Can you work these out from the model? Positions are in its coordinate system, mm. A direction names the side the tool comes from. Round coordinates to 2 decimals unless told otherwise and drop trailing zeros. Loops run counter-clockwise (first coordinate to the right, second up) from the corner with the lowest first, then second, coordinate; pieces in that order, holes last. Notation, with made-up numbers: M 45,1.25 L 74,1.25 A8 cw 74,15.25 Z; hole C 13.5,17 d1. An arc over 180 degrees is marked long. Return JSON: item names as keys, results as strings.
```python
from build123d import *

# Parameters (mm, degrees)
SKETCH3_R               = 14
SKETCH3_R_2             = 6.35
SKETCH3_R_3             = 20
SKETCH3_R_4             = 9.5
BOSS_EXTRUDE6_DEPTH     = 26.5
CUT_EXTRUDE5_START      = 7
SKETCH7_W               = 38
SKETCH7_H               = 71.155333985
CUT_EXTRUDE5_DEPTH      = 12.5
CUT_EXTRUDE6_DEPTH      = 93.278112248
CUT_EXTRUDE6_DEPTH_BACK = 6
CUT_EXTRUDE8_DEPTH      = 93.278112248
CUT_EXTRUDE8_DEPTH_BACK = 6
CUT_EXTRUDE10_DEPTH     = 5
CUT_EXTRUDE10_TAPER     = 5
CUT_EXTRUDE11_DEPTH     = 5
CUT_EXTRUDE11_DRAFT     = -5


with BuildPart() as part:
    # Sketch3 → Boss-Extrude6 (new body)
    # profile 1 of 3: a face of its own
    with BuildSketch(Plane.XY):
        with BuildLine():
            ThreePointArc((0.870489571, 49), (-12.127650844, 35.035893248), (-26.986121482, 47.001417973))
            Line((-26.986121482, 47.001417973), (-19.795158647, -2.855117182))
            ThreePointArc((-19.795158647, -2.855117182), (-1.431227978, 19.948723931), (20, 0))
            ThreePointArc((20, 0), (14.142135624, -14.142135624), (0, -20))
            Line((0, -20), (62, -20))
            Line((62, -20), (62, -8.5))
            Line((62, -8.5), (40, -8.5))
            ThreePointArc((40, -8.5), (33.5, -2), (40, 4.5))
            Line((40, 4.5), (62, 4.5))
            Line((62, 4.5), (62, 16))
            ThreePointArc((62, 16), (24.979840385, 26.107737846), (-0.421043253, 54.873232673))
            ThreePointArc((-0.421043253, 54.873232673), (0.543794593, 52.006780632), (0.870489571, 49))
        make_face()
    # profile 2 of 3: a face of its own
    with BuildSketch(Plane.XY):
        with Locations((-13.129510429, 49)):
            Circle(SKETCH3_R)
        with Locations((-13.129510429, 49)):
            Circle(SKETCH3_R_2, mode=Mode.SUBTRACT)
    # profile 3 of 3: a face of its own
    with BuildSketch(Plane.XY):
        Circle(SKETCH3_R_3)
        Circle(SKETCH3_R_4, mode=Mode.SUBTRACT)
    extrude(amount=BOSS_EXTRUDE6_DEPTH)

    # Sketch7 → Cut-Extrude5 (cut)
    with BuildSketch(Plane.XY.offset(CUT_EXTRUDE5_START)):
        with Locations((43, 15.577666993)):
            Rectangle(SKETCH7_W, SKETCH7_H)
    extrude(amount=CUT_EXTRUDE5_DEPTH, mode=Mode.SUBTRACT)

    # Sketch8 → Cut-Extrude6 (cut, two sides: drawn at the far end of the back side and taken through both)
    with BuildSketch(Plane.XY.offset(26.5).offset(-CUT_EXTRUDE6_DEPTH_BACK)):
        with BuildLine():
            Line((-191.908254211, 170.560932392), (-25.15238927, 34.287747135))
            ThreePointArc((-25.15238927, 34.287747135), (-9.427586496, 30.364127088), (3.603690102, 40))
            Line((3.603690102, 40), (9.001095845, 40))
            Line((9.001095845, 40), (224.356382551, 40))
            Line((224.356382551, 40), (353.256649812, 450.969973536))
            Line((353.256649812, 450.969973536), (-63.007986949, 581.530905928))
            Line((-63.007986949, 581.530905928), (-191.908254211, 170.560932392))
        make_face()
    extrude(amount=CUT_EXTRUDE6_DEPTH + CUT_EXTRUDE6_DEPTH_BACK, mode=Mode.SUBTRACT)

    # Sketch9 → Cut-Extrude8 (cut, two sides: drawn at the far end of the back side and taken through both)
    with BuildSketch(Plane(origin=(0, 0, 0), x_dir=(-1, 0, 0), z_dir=(0, 0, -1)).offset(-CUT_EXTRUDE8_DEPTH_BACK)):
        with BuildLine():
            Line((191.908254211, 170.560932392), (25.15238927, 34.287747135))
            ThreePointArc((25.15238927, 34.287747135), (9.427586496, 30.364127088), (-3.603690102, 40))
            Line((-3.603690102, 40), (-9.001095845, 40))
            Line((-9.001095845, 40), (-224.356382551, 40))
            Line((-224.356382551, 40), (-353.256649812, 450.969973536))
            Line((-353.256649812, 450.969973536), (63.007986949, 581.530905928))
            Line((63.007986949, 581.530905928), (191.908254211, 170.560932392))
        make_face()
    extrude(amount=CUT_EXTRUDE8_DEPTH + CUT_EXTRUDE8_DEPTH_BACK, mode=Mode.SUBTRACT)

    # Sketch11 → Cut-Extrude10 (cut)
    with BuildSketch(Plane.XY):
        with BuildLine():
            Line((8.074790236, 38), (4.759033391, 38))
            ThreePointArc((4.759033391, 38), (-7.381776563, 28.801892282), (-22.54639569, 30.229750349))
            Line((-22.54639569, 30.229750349), (-17.815642783, -2.569605464))
            ThreePointArc((-17.815642783, -2.569605464), (-11.784462263, -13.606118079), (0, -18))
            Line((0, -18), (60, -18))
            Line((60, -18), (60, -10.5))
            Line((60, -10.5), (40, -10.5))
            ThreePointArc((40, -10.5), (31.5, -2), (40, 6.5))
            Line((40, 6.5), (60, 6.5))
            Line((60, 6.5), (60, 13.981994332))
            ThreePointArc((60, 13.981994332), (31.430822369, 20.355773383), (8.074790236, 38))
        make_face()
    extrude(amount=CUT_EXTRUDE10_DEPTH, taper=CUT_EXTRUDE10_TAPER, mode=Mode.SUBTRACT)


with BuildPart() as cut_extrude11_tool:
    # Sketch12 → Cut-Extrude11 (with draft: the straight prism first)
    with BuildSketch(Plane.XY.offset(26.5)):
        with BuildLine():
            Line((8.074790236, 38), (4.759033391, 38))
            ThreePointArc((4.759033391, 38), (-7.381776563, 28.801892282), (-22.54639569, 30.229750349))
            Line((-22.54639569, 30.229750349), (-17.815642783, -2.569605464))
            ThreePointArc((-17.815642783, -2.569605464), (-11.784462263, -13.606118079), (0, -18))
            Line((0, -18), (60, -18))
            Line((60, -18), (60, -10.5))
            Line((60, -10.5), (40, -10.5))
            ThreePointArc((40, -10.5), (31.5, -2), (40, 6.5))
            Line((40, 6.5), (60, 6.5))
            Line((60, 6.5), (60, 13.981994332))
            ThreePointArc((60, 13.981994332), (31.430822369, 20.355773383), (8.074790236, 38))
        make_face()
    extrude(amount=-CUT_EXTRUDE11_DEPTH)
    # Cut-Extrude11: the draft: its side faces are tilted about the plane it starts from
    cut_extrude11_sides = [cut_extrude11_tool.faces().sort_by_distance(p)[0] for p in [
        (31.430822369, 20.355773383, 24),
        (6.416911814, 38, 24),
        (-7.381776563, 28.801892282, 24),
        (-20.181019237, 13.830072443, 24),
        (-11.784462263, -13.606118079, 24),
        (30, -18, 24),
        (60, -14.25, 24),
        (50, -10.5, 24),
        (31.5, -2, 24),
        (50, 6.5, 24),
        (60, 10.240997166, 24),
    ]]
    draft(cut_extrude11_sides, Plane.XY.offset(26.5), CUT_EXTRUDE11_DRAFT)


with BuildPart() as part_1:
    add(part.part)

    # Cut-Extrude11: cut by cut_extrude11_tool
    add(cut_extrude11_tool.part, mode=Mode.SUBTRACT)


solid = part_1.part
```
Q1. Thinking about a two-plate mould opening in Y: for faces 1 (the flat face through (-23.44, 22.42, 13.06)), 2 (the conical face through (-7.11, 28.65, 2.54)), 3 (the flat face through (34, 4, 7)), which applies, pulls with the +Y half, pulls with the -Y half, needs draft (parallel to the pull), parting line crosses it, or undercut?
Results:
{"face 1": "pulls with the -Y half", "face 2": "undercut", "face 3": "needs draft"}
Q2. Suppose I cut it at A-A, the plane z = 17.75. Please give me the cut outline in (x, y).
Results:
{"outline": "M -26.99,47 L -19.8,-2.86 A20 ccw 0,-20 L 24,-20 L 24,26.73 A67 cw -0.42,54.87 A14 ccw Z; hole C -13.13,49 d12.7; hole C 0,0 d19"}
Q3. Suppose I cut it at C-C, the plane z = 23.75. Please give me the cut outline in (x, y), plus the area to 3 significant figures.
Results:
{"outline": "M -25.15,34.29 L -19.8,-2.86 A20 ccw 0,-20 L 62,-20 L 62,-8.5 L 40,-8.5 A6.5 cw 40,4.5 L 62,4.5 L 62,16 A67 cw 9,40 L 3.6,40 A19 cw Z; hole M -22.24,29.81 L -17.58,-2.54 A17.76 ccw 0,-17.76 L 59.76,-17.76 L 59.76,-10.74 L 40,-10.74 A8.74 cw 40,6.74 L 59.76,6.74 L 59.76,13.74 A69.24 cw 7.96,37.76 L 4.89,37.76 A21.24 cw Z", "area": "679 mm2"}
Q4. Suppose I cut it at D-D, the plane x = 50. State how many separate pieces and enclosed holes the cut face has, plus the area to 3 significant figures.
Results:
{"separate pieces": "4", "enclosed holes": "0", "area": "184 mm2"}
Q5. I'm going to push flat-ended pins straight in: pin 1 Ø10 at (x, y) = (-17, 47.5) entering from -Z; pin 2 Ø1.6 at (x, z) = (7.5, 24) entering from +Y; pin 3 Ø6 at (y, z) = (12.5, 15) entering from +X; pin 4 Ø11.5 at (x, y) = (34.5, 0) entering from +Z. Where does each tip first touch, or does it pass through?
Results:
{"pin 1": "stops at z = 6", "pin 2": "stops at y = 40", "pin 3": "stops at x = 24", "pin 4": "stops at z = 26.5"}
Q6. On a 3-axis mill with a long thin cutter (end or side, diameter ignored), from which of +Z, -Z, +X, -X, +Y, -Y can I reach the whole of each face in a straight line? I mean faces 4 (the flat face through (29.58, -17.784, 24.035)), 5 (the flat face through (6, 40, 3)), 6 (the flat face through (30.42, -17.784, 2.465)). Say none if no direction works.
Results:
{"face 4": "+Z", "face 5": "-Z, +X, -X, +Y", "face 6": "-Z"}
Q7. If I drill on line 1 along Y through (x, z) = (5, 8.5); line 2 along Y through (x, z) = (0, 9); line 3 along X through (y, z) = (0, 12.25), over which ranges is the centre line in solid material (lowest first)?
Results:
{"line 1": "y = -20 to -8.08, 8.08 to 45.3", "line 2": "y = -20 to -9.5, 9.5 to 53.98", "line 3": "x = -20.21 to -9.5, 9.5 to 24"}
Q8. Suppose I cut it at B-B, the plane y = 49. Please give me the cut outline in (x, z).
Results:
{"outline": "M -27.13,6 L -19.48,6 L -19.48,20.5 L -27.13,20.5 Z; M -6.78,6 L 2.65,6 L 2.65,20.5 L -6.78,20.5 Z"}
